For this review, take the finished solid that the model builds, in its own axes (mm). Give positions to 0.01 mm unless a question says otherwise; leave off trailing zeros. Loops run counter-clockwise (first coordinate to the right, second up) from the corner with the lowest first, then second, coordinate; pieces in that order, holes last.
```python
from build123d import *

# Parameters (mm, degrees)
SKETCH_2_W                 = 50
SKETCH_2_H                 = 80
EXTRUDE_1_DEPTH            = 10
SKETCH_3_R                 = 3.5
SKETCH_3_R_2               = 3
CUT_EXTRUDE_1_DEPTH        = 49.218253805
MIRROR_2_COPY_1_SKETCH_R   = 3.5
MIRROR_2_COPY_1_SKETCH_R_2 = 3
MIRROR_2_COPY_1_DEPTH      = 49.218253805
FILLET_1_R                 = 2.5


with BuildPart() as part:
    # 草图2 → 凸台-拉伸1 (new body)
    with BuildSketch(Plane.XY):
        Rectangle(SKETCH_2_W, SKETCH_2_H)
    extrude(amount=EXTRUDE_1_DEPTH)

    # 草图3 → 切除-拉伸1 (cut, through all)
    with BuildSketch(Plane(origin=(0, 0, 0), x_dir=(-1, 0, 0), z_dir=(0, 0, -1))):
        with Locations((16.5, 29)):
            Circle(SKETCH_3_R)
        with Locations((16.5, 16.5)):
            Circle(SKETCH_3_R_2)
    cut_extrude_1 = extrude(amount=-CUT_EXTRUDE_1_DEPTH, mode=Mode.SUBTRACT)

    # 镜向1: 切除-拉伸1 across plane
    add(cut_extrude_1.mirror(Plane(origin=(0, 0, 0), x_dir=(0, 0, 1), z_dir=(1, 0, 0))), mode=Mode.SUBTRACT)

    # 镜向2: 切除-拉伸1 across plane
    add(cut_extrude_1.mirror(Plane.ZX), mode=Mode.SUBTRACT)

    # 镜向2 copy 1 sketch → 镜向2 copy 1 (cut, through all)
    with BuildSketch(Plane(origin=(0, 0, 0), x_dir=(1, 0, 0), z_dir=(0, 0, -1))):
        with Locations((16.5, 29)):
            Circle(MIRROR_2_COPY_1_SKETCH_R)
        with Locations((16.5, 16.5)):
            Circle(MIRROR_2_COPY_1_SKETCH_R_2)
    extrude(amount=-MIRROR_2_COPY_1_DEPTH, mode=Mode.SUBTRACT)

    # 圆角1
    fillet_1_edges = [part.edges().sort_by_distance(p)[0] for p in [
        (-25, 40, 5),
        (25, 40, 5),
        (25, -40, 5),
        (-25, -40, 5),
    ]]
    fillet(fillet_1_edges, radius=FILLET_1_R)


solid = part.part
```
Item 1: Take a section at D-D on y = -16.5. Give the boundary of the cut face in (x, z), and give its area (3 significant figures).
Answer:
outline: (-25, 0) - (-19.5, 0) - (-19.5, 10) - (-25, 10) - close; (-13.5, 0) - (13.5, 0) - (13.5, 10) - (-13.5, 10) - close; (19.5, 0) - (25, 0) - (25, 10) - (19.5, 10) - close
area: 380 mm2
Item 2: Take a section at B-B on x = 16.5. Give the boundary of the cut face in (y, z).
Answer:
outline: (-40, 0) - (-32.5, 0) - (-32.5, 10) - (-40, 10) - close; (-25.5, 0) - (-19.5, 0) - (-19.5, 10) - (-25.5, 10) - close; (-13.5, 0) - (13.5, 0) - (13.5, 10) - (-13.5, 10) - close; (19.5, 0) - (25.5, 0) - (25.5, 10) - (19.5, 10) - close; (32.5, 0) - (40, 0) - (40, 10) - (32.5, 10) - close
Item 3: Take a section at C-C on z = 5.5. State how many separate pieces and enclosed holes the cut face has, and give its area (3 significant figures).
Answer:
separate pieces: 1
enclosed holes: 8
area: 3,730 mm2
Item 4: Take a section at A-A on y = 29. Give the boundary of the cut face in (x, z).
Answer:
outline: (-25, 0) - (-20, 0) - (-20, 10) - (-25, 10) - close; (-13, 0) - (13, 0) - (13, 10) - (-13, 10) - close; (20, 0) - (25, 0) - (25, 10) - (20, 10) - close
Item 5: The part is to be moulded in two halves that separate along Y. For faces 1 (the flat face through (0, 1, 10)), 2 (the cylindrical face through (-24.287, 39.248, 5.07)), 3 (the cylindrical face through (-14.1, -14.7, 4.9)), 4 (the cylindrical face through (16.04, 32.47, 4.93)), say which applies: released by +Y, released by -Y, zero draft, split by the parting line, or undercut.
Answer:
face 1: zero draft
face 2: released by +Y
face 3: undercut
face 4: undercut
Item 6: For L1, parallel to Y at x = -16.5, z = 7; L2, parallel to X at y = -29, z = 5; L3, parallel to Y at x = 19, z = 8.75, list the stretches that pass through material, from the lowest coordinate up.
Answer:
L1: y = -40 to -32.5, -25.5 to -19.5, -13.5 to 13.5, 19.5 to 25.5, 32.5 to 40
L2: x = -25 to -20, -13 to 13, 20 to 25
L3: y = -40 to -31.45, -26.55 to -18.16, -14.84 to 14.84, 18.16 to 26.55, 31.45 to 40
